Input: part model. Units: mm. Frame: model coordinates. Give positions to 0.01 mm unless a question says otherwise; leave off trailing zeros. Loops run counter-clockwise (first coordinate to the right, second up) from the corner with the lowest first, then second, coordinate; pieces in that order, holes last. Notation, with made-up numbers: (87.25, 79) - (116.25, 79) arc R7 ccw to (116.25, 92) - close; hole circle Ø3 at (74, 43). An arc over 180 degrees is marked (long way). Answer as a JSON object with one key per item and string values. Group by question number.
(1) Material intervals for L1, parallel to Z at x = 0.2, y = -14.5; L2, parallel to Z at x = 0.3, y = -22; L3, parallel to Y at x = 2.6, z = 73, sorted ascending.
(2) Section query C-C (z = -132.5). Return loops of the section in (x, y).
(3) Section query A-A (z = 78). Return loops of the section in (x, y).
(4) Section query B-B (x = 0.5). Return loops of the section in (y, z), plus the area to 3 significant figures.
(5) Pin query (flat end, axial travel): P1, Ø0.9, axis at x = 1, z = -95, coming from the -Y side. Return the tip coordinate at first contact, or that it passes through.
Autodesk Inventor part; units mm, degrees
ref_plane "YZ Plane" through (0, 0, 0) normal (1, 0, 0) x (0, 1, 0)
ref_plane "XZ Plane" through (0, 0, 0) normal (0, 1, 0) x (-1, 0, 0)
ref_plane "XY Plane" through (0, 0, 0) normal (0, 0, 1) x (1, 0, 0)
sketch "스케치1" plane through (0, 0, 0) normal (1, 0, 0) x (0, 1, 0)
  line L0 (30, 195) -> (-30, 195)
  line L1 (-30, 195) -> (-30, -195)
  line L2 (-30, -195) -> (30, -195)
  line L3 (30, -195) -> (30, 195)
  point P0 (0, 0)
  dimension "d0" = 60
  dimension "d1" = 390
  dimension "d2" = 30
  dimension "d3" = 195
extrude "돌출1" add sketch "스케치1" along normal blind 3
sketch "스케치2" plane through (3, 0, 0) normal (1, 0, 0) x (0, 0, -1)
  line L0 (-195, -30) -> (195, -30)
  line L1 (-145, -30) -> (-25, -30)
  line L2 (-25, -30) -> (-25, -10)
  line L3 (-25, -10) -> (-145, -10)
  line L4 (-145, -10) -> (-145, -30)
  line L5 (-195, 30) -> (-195, -30)
  line L6 (0, 0) -> (0, -66.648) construction
  line L7 (25, -10) -> (145, -10)
  line L8 (145, -10) -> (145, -30)
  line L9 (145, -30) -> (25, -30)
  line L10 (25, -30) -> (25, -10)
  line L11 (195, -30) -> (195, 30)
  dimension "d6" = 20
  dimension "d7" = 50
  dimension "d8" = 25
  dimension "d9" = 50
  dimension "d10" = 25
  dimension "d11" = 20
extrude "돌출2" cut sketch "스케치2" against normal through all
sketch "스케치3" plane through (3, 0, 0) normal (1, 0, 0) x (0, 0, -1)
  line L0 (-170, 132.4891) -> (-170, -92.5)
  line L1 (0, 133.9107) -> (0, -104.4082)
  line L2 (170, 113.5044) -> (170, -115.928)
  line L3 (195, -30) -> (195, 30)
  line L4 (-195, 30) -> (-195, -30)
  line L5 (-170, -22) -> (-170, -18) construction
  line L6 (-168, -22) -> (-168, -18)
  line L7 (-172, -18) -> (-172, -22)
  arc A0 (-172, -22) -> (-168, -22) centre (-170, -22) ccw
  arc A1 (-168, -18) -> (-172, -18) centre (-170, -18) ccw
  line L8 (0, -22) -> (0, -18) construction
  line L9 (2, -22) -> (2, -18)
  line L10 (-2, -18) -> (-2, -22)
  arc A2 (-2, -22) -> (2, -22) centre (0, -22) ccw
  arc A3 (2, -18) -> (-2, -18) centre (0, -18) ccw
  line L11 (170, -22) -> (170, -18) construction
  line L12 (172, -22) -> (172, -18)
  line L13 (168, -18) -> (168, -22)
  arc A4 (168, -22) -> (172, -22) centre (170, -22) ccw
  arc A5 (172, -18) -> (168, -18) centre (170, -18) ccw
  line L14 (145, -30) -> (195, -30)
  line L15 (-25, -30) -> (25, -30)
  line L16 (-195, -30) -> (-145, -30)
  line L17 (-120, 10) -> (-40, 10)
  line L18 (-40, 10) -> (-40, 13)
  line L19 (-40, 13) -> (-120, 13)
  line L20 (-120, 13) -> (-120, 10)
  point P0 (0, 0)
  point P1 (-170, -20)
  point P2 (0, -20)
  point P3 (170, -20)
  dimension "d14" = 25
  dimension "d15" = 25
  dimension "d16" = 0
  dimension "d17" = 4
  dimension "d18" = 4
  dimension "d19" = 4
  dimension "d20" = 4
  dimension "d21" = 4
  dimension "d22" = 4
  dimension "d23" = 10
  dimension "d24" = 10
  dimension "d25" = 10
  dimension "d36" = 80
  dimension "d37" = 3
  dimension "d38" = 75
  dimension "d39" = 10
extrude "돌출3" cut sketch "스케치3" against normal blind 10
equation "\"d6\" = d11"
equation "\"d10\" = d8"
properties part number "라즈베리파이보관_옆판" material "PMMA 플라스틱"
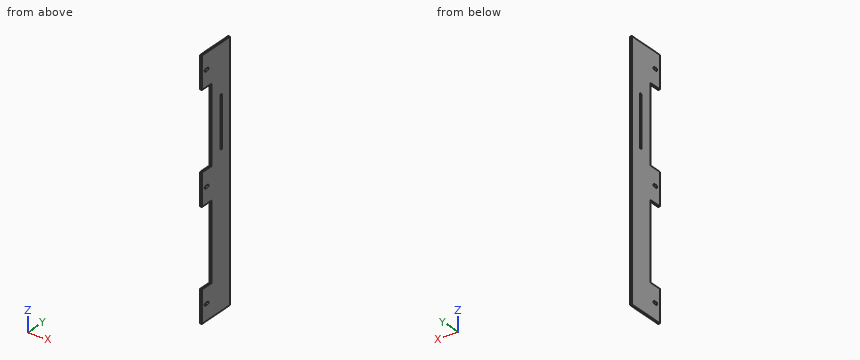
Recorded:
{
 "1": {"L1": "z = -195 to -145, -25 to 25, 145 to 195", "L2": "z = -195 to -172, -168 to -145, -25 to -2, 2 to 25, 145 to 168, 172 to 195", "L3": "y = -10 to 10, 13 to 30"},
 "2": {"outline": "(0, -10) - (3, -10) - (3, 30) - (0, 30) - close"},
 "3": {"outline": "(0, -10) - (3, -10) - (3, 10) - (0, 10) - close; (0, 13) - (3, 13) - (3, 30) - (0, 30) - close"},
 "4": {"outline": "(-30, -195) - (30, -195) - (30, 195) - (-30, 195) - (-30, 145) - (-10, 145) - (-10, 25) - (-30, 25) - (-30, -25) - (-10, -25) - (-10, -145) - (-30, -145) - close; hole (-22, -172) - (-18, -172) arc R2 ccw to (-18, -168) - (-22, -168) arc R2 ccw to start; hole (-22, -2) - (-18, -2) arc R2 ccw to (-18, 2) - (-22, 2) arc R2 ccw to start; hole (-22, 168) - (-18, 168) arc R2 ccw to (-18, 172) - (-22, 172) arc R2 ccw to start; hole (10, 40) - (13, 40) - (13, 120) - (10, 120) - close", "area": "18,300 mm^2"},
 "5": {"P1": "stops at y = -10"}
}
